from build123d import *

# Parameters (mm, degrees)
CYLINDER001_R     = 1
CYLINDER001_DEPTH = 50
CYLINDER_R        = 1
CYLINDER_DEPTH    = 50
ARRAY_Y_COUNT     = 2
ARRAY_Y_PITCH     = 10
BOX_W             = 10
BOX_H             = 22
BOX_DEPTH         = 18


with BuildPart() as cylinder001:
    # Cylinder001 → Cylinder001 (new body)
    with BuildSketch(Plane(origin=(-10, 11, 14), x_dir=(0, 0, -1), z_dir=(1, 0, 0))):
        Circle(CYLINDER001_R)
    extrude(amount=CYLINDER001_DEPTH)


with BuildPart() as fusion:
    # Cylinder → Cylinder (new body)
    with BuildSketch(Plane.XY.offset(-10)):
        Circle(CYLINDER_R)
    extrude(amount=CYLINDER_DEPTH)

    # Array Y: Fusion ×2


with BuildPart() as fusion_1:
    add(fusion.part)
    with Locations(*[(0, i * ARRAY_Y_PITCH, 0) for i in range(1, ARRAY_Y_COUNT)]):
        add(fusion.part)


with BuildPart() as fusion_2:
    # Array placement: moved
    add(fusion_1.part.moved(Location((6, 6, 0))))

    # Fusion: union Cylinder001
    add(cylinder001.part)


with BuildPart() as cut:
    # Box → Box (new body)
    with BuildSketch(Plane.XY):
        with Locations((5, 11)):
            Rectangle(BOX_W, BOX_H)
    extrude(amount=BOX_DEPTH)

    # Cut: cut Fusion
    add(fusion_2.part, mode=Mode.SUBTRACT)


solid = cut.part
Check sheet for the modelled part. Datum: model origin and axes. Units: mm. Round coordinates to 2 decimals unless told otherwise and drop trailing zeros. Write each loop counter-clockwise with the first axis right and the second up, starting at its lowest first coordinate (ties: lowest second). Pieces come first, ordered by that corner, then holes. Notation, with made-up numbers: (-5, 47.25) -> (10, 47.25) arc R21 cw to (10, 74.25) -> close; hole circle Ø10 at (58.25, -6.75). An arc over 180 degrees is marked (long way). Answer as CSV lines item,"result". Start each with the question number.
1) Section check C-C on z = 14. Enter the section's corners in (x, y).
2) Release check for a two-part mould opening along Y. For faces 1 (the flat face through (5, 22, 9)), 2 (the flat face through (5, 0, 9)), 3 (the flat face through (0, 11, 9)), 4 (the cylindrical face through (6, 15, 9)) record: pulls with the +Y half, pulls with the -Y half, needs draft (parallel to the pull), parting line crosses it, or undercut.
3) Section check D-D on y = 16. Enter the section's corners in (x, z).
4) Section check A-A on x = 6. Enter the section's corners in (y, z).
5) Material ranges on line 1 (Y direction, x = 6, z = 9.75); line 2 (X direction, y = 6, z = 6.5); line 3 (Y direction, x = 4.5, z = 14), recorded low to high. Write a range as from..to.
6) Section check B-B on y = 11. Enter the section's corners in (x, z), and give its area (3 significant figures).
Found:
1,outline,"(0, 0) -> (10, 0) -> (10, 10) -> (0, 10) -> close; (0, 12) -> (10, 12) -> (10, 22) -> (0, 22) -> close; hole circle Ø2 at (6, 6); hole circle Ø2 at (6, 16)"
2,face 1,"pulls with the +Y half"
2,face 2,"pulls with the -Y half"
2,face 3,"needs draft"
2,face 4,"undercut"
3,outline,"(0, 0) -> (5, 0) -> (5, 18) -> (0, 18) -> close; (7, 0) -> (10, 0) -> (10, 18) -> (7, 18) -> close"
4,outline,"(0, 0) -> (5, 0) -> (5, 18) -> (0, 18) -> close; (7, 0) -> (15, 0) -> (15, 18) -> (7, 18) -> close; (17, 0) -> (22, 0) -> (22, 18) -> (17, 18) -> close; hole circle Ø2 at (11, 14)"
5,line 1,"y = 0..5, 7..15, 17..22"
5,line 2,"x = 0..5, 7..10"
5,line 3,"y = 0..10, 12..22"
6,outline,"(0, 0) -> (10, 0) -> (10, 13) -> (0, 13) -> close; (0, 15) -> (10, 15) -> (10, 18) -> (0, 18) -> close"
6,area,"160 mm^2"
